from build123d import *

# Parameters (mm, degrees)
SKETCH1_R           = 10
SKETCH1_R_2         = 3
BOSS_EXTRUDE1_DEPTH = 6
FILLET1_R           = 10


with BuildPart() as part:
    # Sketch1 → Boss-Extrude1 (new body)
    with BuildSketch(Plane.XY):
        with BuildLine():
            Line((15, 174.355957742), (15, -174.355957742))
            ThreePointArc((15, -174.355957742), (-175, 0), (15, 174.355957742))
        make_face()
        with Locations((0, 120)):
            Circle(SKETCH1_R, mode=Mode.SUBTRACT)
        with Locations((0, -155)):
            Circle(SKETCH1_R_2, mode=Mode.SUBTRACT)
    extrude(amount=BOSS_EXTRUDE1_DEPTH)

    # Fillet1
    fillet1_edges = [part.edges().sort_by_distance(p)[0] for p in [
        (15, 174.355957742, 3),
        (15, -174.355957742, 3),
    ]]
    fillet(fillet1_edges, radius=FILLET1_R)


solid = part.part
Check sheet for the modelled part. Datum: model origin and axes. Units: mm. Give positions to 0.01 mm unless a question says otherwise; leave off trailing zeros. Loops run counter-clockwise (first coordinate to the right, second up) from the corner with the lowest first, then second, coordinate; pieces in that order, holes last. Notation, with made-up numbers: M 77,50 L 109,50 A15 cw 109,77 Z; hole C 74.5,28 d4. An arc over 180 degrees is marked long. Answer as a JSON object with one key per item and string values. Group by question number.
Q1. Go/stop test with a flat-tipped pin: P1, Ø2, axis at x = -125.5, y = -124, coming from the -Z side. Record where the tip stops, or that it passes through.
Q2. Cross-section at A-A on y = 120. Record the cut outline in (x, z).
Q3. Material ranges on line 1 along Y through (x, z) = (0, 2.6); line 2 along X through (y, z) = (-155, 2.75); line 3 along X through (y, z) = (15, 2.5), recorded low to high. Write a range as [from, to].
Q4. Cross-section at B-B on z = 2.75. Record the cut outline in (x, y), then the cut area to 3 significant figures.
Q5. Release check for a two-part mould opening along X. For faces 1 (the flat face through (-58, 2, 6)), 2 (the cylindrical face through (12.25, 171.81, 3.04)), 3 (the cylindrical face through (1.61, -152.47, 2.96)) record: released by +X, released by -X, zero draft, split by the parting line, or undercut.
Q6. Cross-section at C-C on y = -113.5. Record the cut outline in (x, z).
Q7. Cross-section at D-D on x = -163. Record the cut outline in (y, z).
Evaluation:
{
 "1": {"P1": "passes through"},
 "2": {"outline": "M -127.38,0 L -10,0 L -10,6 L -127.38,6 Z; M 10,0 L 15,0 L 15,6 L 10,6 Z"},
 "3": {"line 1": "y = [-175, -158], [-152, 110], [130, 175]", "line 2": "x = [-81.24, -3], [3, 15]", "line 3": "x = [-174.36, 15]"},
 "4": {"outline": "M 5.3,-174.92 A10 ccw 15,-164.92 L 15,164.92 A10 ccw 5.3,174.92 A175 ccw long Z; hole C 0,120 d20; hole C 0,-155 d6", "area": "53,000 mm2"},
 "5": {"face 1": "zero draft", "face 2": "released by +X", "face 3": "undercut"},
 "6": {"outline": "M -133.2,0 L 15,0 L 15,6 L -133.2,6 Z"},
 "7": {"outline": "M -63.69,0 L 63.69,0 L 63.69,6 L -63.69,6 Z"}
}
